Geometry check sheet. Reference: the model listing, model coordinates, mm. Face numbers are marked on the shaded views. A direction names the side the tool comes from. Give positions to 0.01 mm unless a question says otherwise; leave off trailing zeros. Order: outer loops, then holes, each group sorted by start corner. A loop starts at its lowest first (then second) coordinate and runs counter-clockwise, first axis right, second up. Notation, with made-up numbers: M -27,73 L 15,73 A24 cw 15,90 Z; hole C 18,65 d9. An arc over 180 degrees is marked long. Answer as CSV lines item,"result".
from build123d import *

# Parameters (mm, degrees)
SALIENTE_EXTRUIR1_DEPTH = 5
SALIENTE_EXTRUIR2_DEPTH = 40
EXTRUIR_L_MINA2_REACH   = 62.374
CROQUIS5_W              = 75.430750805
CROQUIS5_H              = 6
REDONDEO1_R             = 5
CROQUIS6_R              = 3
CORTAR_EXTRUIR1_DEPTH   = 40


with BuildPart() as part:
    # Croquis1 → Saliente-Extruir1 (new body)
    with BuildSketch(Plane.XY):
        with BuildLine():
            Line((-25, 16.317101546), (-95, 16.317101546))
            Line((-95, 16.317101546), (-95, 1.317101546))
            Line((-95, 1.317101546), (-25, 1.317101546))
            Line((-25, 1.317101546), (-25, -21.182898454))
            Line((-25, -21.182898454), (30, -21.182898454))
            ThreePointArc((30, -21.182898454), (31.913417162, -20.802296117), (33.535533906, -19.71843236))
            Line((33.535533906, -19.71843236), (-23.535533906, 37.352635452))
            ThreePointArc((-23.535533906, 37.352635452), (-24.619397663, 35.730518707), (-25, 33.817101546))
            Line((-25, 33.817101546), (-25, 16.317101546))
        make_face()
    extrude(amount=SALIENTE_EXTRUIR1_DEPTH)

    # Croquis2 → Saliente-Extruir2 (add)
    with BuildSketch(Plane.XY.offset(5)):
        with BuildLine():
            Line((-4.545941546, 18.363043092), (-9.495689014, 23.31279056))
            ThreePointArc((-9.495689014, 23.31279056), (-9.495689014, -5.678587469), (19.495689014, -5.678587469))
            Line((19.495689014, -5.678587469), (14.545941546, -0.72884))
            ThreePointArc((14.545941546, -0.72884), (-4.545941546, -0.72884), (-4.545941546, 18.363043092))
        make_face()
    extrude(amount=SALIENTE_EXTRUIR2_DEPTH)

    # Croquis5 → Extruir-Lámina2 (add, up to next)
    with BuildSketch(Plane(origin=(-21.625922377, 0, 38.118018916), x_dir=(0.869770425, 0, 0.493456592), z_dir=(-0.493456592, 0, 0.869770425)), mode=Mode.PRIVATE) as extruir_l_mina2_sk1:
        with Locations((-29.252830647, 6.317101546)):
            Rectangle(CROQUIS5_W, CROQUIS5_H)
    extruir_l_mina2_tool1 = extrude(extruir_l_mina2_sk1.sketch, amount=-EXTRUIR_L_MINA2_REACH, mode=Mode.PRIVATE) - part.part
    add(extruir_l_mina2_tool1.solids().sort_by_distance((-47.069169, 6.317102, 23.683017))[0])

    # Redondeo1
    redondeo1_edges = [part.edges().sort_by_distance(p)[0] for p in [
        (-95, 1.317101546, 2.5),
        (-95, 16.317101546, 2.5),
        (-25, -21.182898454, 2.5),
    ]]
    fillet(redondeo1_edges, radius=REDONDEO1_R)

    # Croquis6 → Cortar-Extruir1 (cut)
    with BuildSketch(Plane.XY.offset(5)):
        with Locations((-87.5, 6.317101546)):
            Circle(CROQUIS6_R)
        with Locations((-17.5, -13.682898454)):
            Circle(CROQUIS6_R)
        with Locations((-17.5, 31.317101546)):
            Circle(CROQUIS6_R)
        with Locations((27.5, -13.682898454)):
            Circle(CROQUIS6_R)
    extrude(amount=-CORTAR_EXTRUIR1_DEPTH, mode=Mode.SUBTRACT)


solid = part.part
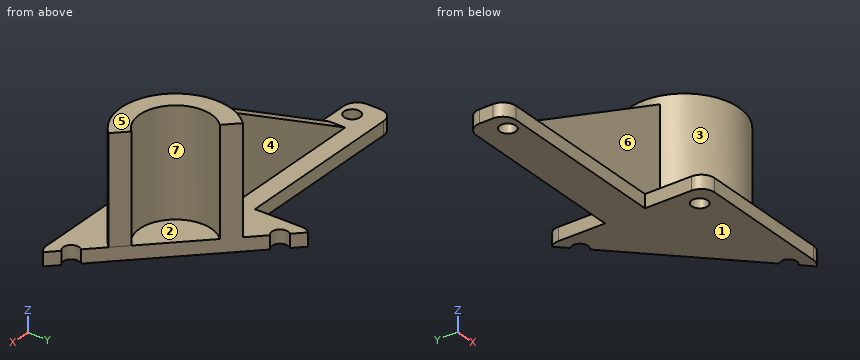
(1) Material ranges on line 1 (Y direction, x = -17.5, z = 3.9); line 2 (Y direction, x = -87.5, z = 4); line 3 (Z direction, x = -80, y = 4), recorded low to high.
The answers:
line 1,"y = -21.18 to -16.68, -10.68 to 28.32"
line 2,"y = 1.32 to 3.32, 9.32 to 16.32"
line 3,"z = 0 to 5"
(2) Section check D-D on x = -68.5. Enter the section's corners in (y, z).
The answers:
outline,"M 1.32,0 L 16.32,0 L 16.32,5 L 9.32,5 L 9.32,11.52 L 3.32,11.52 L 3.32,5 L 1.32,5 Z"
(3) Section check A-A on x = -87.5. Enter the section's corners in (y, z).
The answers:
outline,"M 1.32,0 L 3.32,0 L 3.32,5 L 1.32,5 Z; M 9.32,0 L 16.32,0 L 16.32,5 L 9.32,5 Z"
(4) Tool access check on the marked faces 4, 5, 6 and 7. Record the directions out of +Z, -Z, +X, -X, +Y, -Y that give a thin tool (end or side, any length) a straight path to the whole face; none if there is none.
The answers:
face 4,"+Z, -X, +Y"
face 5,"+Z, +X, -X, +Y, -Y"
face 6,"+Z, -X, -Y"
face 7,"+Z"
(5) Section check C-C on y = 25.5. Enter the section's corners in (x, z), then the cut area to 3 significant figures.
The answers:
outline,"M -25,0 L -11.68,0 L -11.68,5 L -25,5 Z"
area,"66.6 mm2"
(6) Section check B-B on z = 7. Enter the section's corners in (x, y), then the cut area to 3 significant figures.
The answers:
outline,"M -76.47,3.32 L -14.75,3.32 A20.5 ccw 19.5,-5.68 L 14.55,-0.73 A13.5 cw -4.55,18.36 L -9.5,23.31 A20.5 ccw -15.49,9.32 L -76.47,9.32 Z"
area,"741 mm2"
(7) Gauge pin test, flat ends, axial feed: P1, Ø4, axis at y = 24, z = 1.5, coming from the -X side; P2, Ø1.5, axis at x = -43.5, z = 3, coming from the +Y side; P3, Ø4, axis at x = -4.5, z = 29, coming from the -Y side; P4, Ø5, axis at x = -17.5, y = -13.68, coming from the +Z side. Record the tip position at first contact, or that the pin passes through.
The answers:
P1,"stops at x = -25"
P2,"stops at y = 16.32"
P3,"stops at y = -10.26"
P4,"passes through"
(8) Draft check along Y on the marked faces 1, 2 and 3. Enter one of: +Y half, -Y half, draft (parallel to the pull), parting line (faces both ways), or undercut.
The answers:
face 1,"draft"
face 2,"undercut"
face 3,"parting line"
